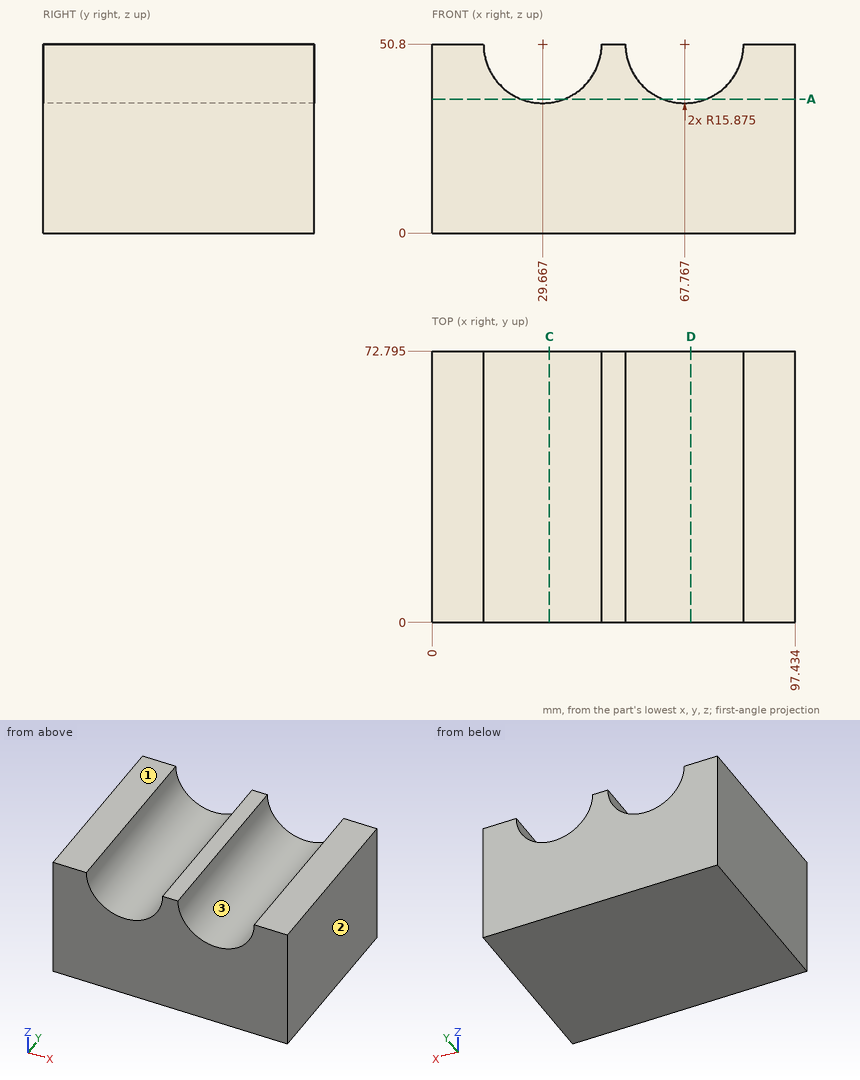
Geometry: see drawing. Coordinates: mm, zero at the bounding-box minimum. Coordinates: 2 decimals unless noted, no trailing zeros. Write each loop counter-clockwise with the first axis right and the second up, starting at its lowest first coordinate (ties: lowest second). Pieces come first, ordered by that corner, then holes. Notation, with made-up numbers: (41.25, -38.5) - (61.25, -38.5) arc R23 cw to (61.25, -23.5) - close; hole circle Ø4 at (39, 0.5). An arc over 180 degrees is marked (long way). Put each result on its own line as item: value. Start each with the question number.
1) Ray query, L1, parallel to X at y = 4, z = 39 (1 decimal); L2, parallel to X at y = 32.5, z = 45.5; L3, parallel to Z at x = 68.5, y = 29.5. Return the intervals inside material, ascending.
2) Cut plane A-A (z = 36). Return the cut outline in (x, y) (1 decimal).
3) Mould query, pull axis X, two halves, no side actions, for the marked faces 1, 2 and 3. Classes: pulls with the +X half, pulls with the -X half, needs draft (parallel to the pull), parting line crosses it, or undercut.
4) Cut plane C-C (x = 31.5). Return the cut outline in (y, z) (1 decimal).
5) Contact query for a flat-ended pin moving along its axis: pin 1 (5 mm diameter, centred on x = 21.5, y = 26.5, fed in from +Z). Output: stop coordinate, or through.
Resolved:
1. L1: x = 0 to 19, 40.3 to 57.1, 78.4 to 97.4
1. L2: x = 0 to 14.7, 44.63 to 52.8, 82.73 to 97.43
1. L3: z = 0 to 34.94
2. outline: (0, 0) - (23.9, 0) - (23.9, 72.8) - (0, 72.8) - close; (35.4, 0) - (62, 0) - (62, 72.8) - (35.4, 72.8) - close; (73.5, 0) - (97.4, 0) - (97.4, 72.8) - (73.5, 72.8) - close
3. face 1: needs draft
3. face 2: pulls with the +X half
3. face 3: undercut
4. outline: (0, 0) - (72.8, 0) - (72.8, 35) - (0, 35) - close
5. pin 1: stops at z = 39.04
